Autodesk Inventor part; units mm, degrees
ref_plane "YZ Plane" through (0, 0, 0) normal (1, 0, 0) x (0, 1, 0)
ref_plane "XZ Plane" through (0, 0, 0) normal (0, 1, 0) x (-1, 0, 0)
ref_plane "XY Plane" through (0, 0, 0) normal (0, 0, 1) x (1, 0, 0)
sketch "Sketch1" plane through (0, 0, 0) normal (0, 0, 1) x (1, 0, 0)
  point P0 (0, 0)
sketch "Sketch2" plane through (0, 0, 0) normal (0, 0, 1) x (1, 0, 0)
  point P0 (0, 0)
sketch "Sketch3" plane through (0, 0, 0) normal (0, 0, 1) x (1, 0, 0)
  line L0 (7.62, 10.922) -> (7.62, 14.351)
  line L1 (7.62, 14.351) -> (-5.08, 14.351)
  line L2 (-5.08, 14.351) -> (-5.08, 10.922)
  line L3 (-5.08, 10.922) -> (-1.27, 10.922)
  line L4 (-1.27, 10.922) -> (-1.27, 6.477)
  line L5 (-1.27, 6.477) -> (-5.08, 6.477)
  line L6 (-5.08, 6.477) -> (-5.08, 2.921)
  line L7 (-5.08, 2.921) -> (-1.27, 2.921)
  line L8 (-1.27, 2.921) -> (-1.27, -1.397)
  line L9 (-1.27, -1.397) -> (3.302, -1.397)
  line L10 (3.302, -1.397) -> (3.302, 2.921)
  line L11 (3.302, 2.921) -> (7.112, 2.921)
  line L12 (7.112, 2.921) -> (7.112, 6.477)
  line L13 (7.112, 6.477) -> (3.302, 6.477)
  line L14 (3.302, 6.477) -> (3.302, 10.922)
  line L15 (3.302, 10.922) -> (7.62, 10.922)
  point P0 (0, 0)
  dimension "d6" = 3.429
  dimension "d7" = 12.7
  dimension "d9" = 3.429
  dimension "d12" = 3.81
  dimension "d13" = 4.445
  dimension "d14" = 3.556
  dimension "d15" = 4.572
  dimension "d16" = 4.318
  dimension "d17" = 3.556
  dimension "d21" = 4.318
extrude "Extrusion1" add sketch "Sketch3" along normal blind 152.4
shell "Shell1" thickness 1.27 removed faces 0
properties part number "RIPnewslide2"
Source: CAD feature listing. Evaluate the final solid. Frame: model axes, mm. A direction names the side the tool comes from. Coordinates: 2 decimals unless noted, no trailing zeros. Loops run counter-clockwise (first coordinate to the right, second up) from the corner with the lowest first, then second, coordinate; pieces in that order, holes last. Notation, with made-up numbers: (15, 29.25) - (45, 29.25) arc R16 ccw to (45, 36.25) - close; hole circle Ø8 at (80, -30). An arc over 180 degrees is marked (long way). Return JSON: item names as keys, results as strings.
Q1. Section B-B, the plane y = 8.25. Return loops of the section in (x, z), plus the area to 3 significant figures.
Results:
{"outline": "(-1.27, 0) - (3.3, 0) - (3.3, 152.4) - (-1.27, 152.4) - close; hole (0, 1.27) - (2.03, 1.27) - (2.03, 151.13) - (0, 151.13) - close", "area": "392 mm2"}
Q2. Mould query, pull axis X, two halves, no side actions, for faces 6 (the flat face through (-1.27, 9, 75)), 7 (the flat face through (3.302, 1, 75)), 8 (the flat face through (-2, 4.191, 75)). Classes: released by +X, released by -X, zero draft, split by the parting line, or undercut.
Results:
{"face 6": "released by -X", "face 7": "released by +X", "face 8": "undercut"}
Q3. Access query for faces 1 (the flat face through (-2, 5.207, 75)), 2 (the flat face through (-3, 6.477, 75)), 3 (the flat face through (5, 6.477, 75)), 4 (the flat face through (-1.27, 1, 75)), 5 (the flat face through (5, 2.921, 75)). Directions: +Z, -Z, +X, -X, +Y, -Y. A direction counts if a zero-diameter tool reaches every point of the face in a straight line with its end or side. Return the directions, or none.
Results:
{"face 1": "none", "face 2": "+Z, -Z, -X", "face 3": "+Z, -Z, +X", "face 4": "+Z, -Z, -X, -Y", "face 5": "+Z, -Z, +X, -Y"}
Q4. Contact query for flat-ended pins moving along their axis: P1, Ø1.3, axis at y = 9.5, z = 91.5, coming from the -X side; P2, Ø3, axis at x = 6, z = 93, coming from the -Y side; P3, Ø3.5, axis at y = 1.5, z = 47, coming from the +X side. Output: stop coordinate, or through.
Results:
{"P1": "x = -1.27", "P2": "y = 2.92", "P3": "x = 7.11"}
Q5. Material intervals for line 1 along Y through (x, z) = (2.75, 40); line 2 along Y through (x, z) = (4.5, 87); line 3 along Y through (x, z) = (6, 18.5), sorted ascending.
Results:
{"line 1": "-1.4 to 4.19, 5.21 to 12.19, 13.08 to 14.35", "line 2": "2.92 to 4.19, 5.21 to 6.48, 10.92 to 12.19, 13.08 to 14.35", "line 3": "2.92 to 6.48, 10.92 to 12.19, 13.08 to 14.35"}
